Read the model definition and answer for the solid it produces. Units are mm, in the model's axes. A direction names the side the tool comes from. Coordinates: 2 decimals unless noted, no trailing zeros. Write each loop counter-clockwise with the first axis right and the second up, starting at its lowest first coordinate (ties: lowest second). Pieces come first, ordered by that corner, then holes.
(1) Given pin 1 (1.5 mm diameter, centred on y = 37, z = -7, fed in from -X); pin 2 (4.5 mm diameter, centred on y = 35.5, z = -2.5, fed in from +X); pin 3 (5 mm diameter, centred on y = 35, z = 0, fed in from +X) (3 decimals); pin 4 (1.5 mm diameter, centred on x = -35.5, y = 24.5, fed in from +Z), each flat-ended and moving along its own axis, determine where each tip first touches the part or whether it passes through.
(2) Which of the six approach directions +Z, -Z, +X, -X, +Y, -Y give full straight-line access (tool end or side, diameter ignored) to faces 1 (the flat face through (-17.091, 22.918, 29.392)), 2 (the flat face through (-11.7, 31.77, 26.73)), 3 (the flat face through (37, 25, 7.5)), 4 (the flat face through (-24.763, 24.86, -27.89)), 5 (the flat face through (29, 32, -3))?
(3) The mould has two halves that part along Z. Classify faces 6 (the flat face through (19.409, 25.887, 33.827)), 7 (the flat face through (-39, 26, 0)), 8 (the flat face through (-31.961, 7.605, 24.226)): +Z half, -Z half, draft (parallel to the pull), parting line (faces both ways), or undercut.
(4) Section A-A on z = 0 is taken. Write down the section's boundary in (x, y).
(5) Section B-B on y = 5 is taken. Write down the section's boundary in (x, z).
(6) Find the intervals of material crossed by probe 1 along Y at (x, z) = (31.5, 0); probe 2 along X at (y, z) = (32, 29.5); probe 3 along X at (y, z) = (38, 6.5), in increasing order.
(7) Section C-C on x = 0 is taken. Write down the section's boundary in (y, z).
from build123d import *

# Parameters (mm, degrees)
SKETCH1_R           = 45
BOSS_EXTRUDE1_DEPTH = 15
CUT_EXTRUDE1_DEPTH  = 66.383484153
CIRPATTERN1_COUNT   = 3
SKETCH4_R           = 4
BOSS_EXTRUDE2_DEPTH = 5
SKETCH6_R           = 7.5
SKETCH6_R_2         = 4
BOSS_EXTRUDE3_DEPTH = 10
CIRPATTERN2_COUNT   = 6


with BuildPart() as part:
    # Sketch1 → Boss-Extrude1 (new body)
    with BuildSketch(Plane(origin=(0, 0, 0), x_dir=(1, 0, 0), z_dir=(0, 1, 0))):
        with Locations(Location((0, 0, 0), (0, 0, 270))):
            Circle(SKETCH1_R)
    extrude(amount=BOSS_EXTRUDE1_DEPTH)

    # Sketch2 → Cut-Extrude1 (cut, through all)
    with BuildSketch(Plane(origin=(0, 15, 0), x_dir=(1, 0, 0), z_dir=(0, 1, 0))):
        with BuildLine():
            Line((-5, 35), (-5, 44.72135955))
            ThreePointArc((-5, 44.72135955), (0, 45), (5, 44.72135955))
            Line((5, 44.72135955), (5, 35))
            ThreePointArc((5, 35), (0, 30), (-5, 35))
        make_face()
    cut_extrude1 = extrude(amount=-CUT_EXTRUDE1_DEPTH, mode=Mode.SUBTRACT)

    # CirPattern1: Cut-Extrude1 ×3 about axis
    cirpattern1_axis = Axis((0, 0, 0), (0, 1, 0))
    for i in range(1, CIRPATTERN1_COUNT):
        add(cut_extrude1.rotate(cirpattern1_axis, i * 360 / CIRPATTERN1_COUNT), mode=Mode.SUBTRACT)

    # Sketch4 → Boss-Extrude2 (add)
    with BuildSketch(Plane(origin=(39, 0, 0), x_dir=(0, 0, -1), z_dir=(1, 0, 0))):
        with BuildLine():
            Line((-7.5, 35), (-7.5, 15))
            Line((-7.5, 15), (7.5, 15))
            Line((7.5, 15), (7.5, 35))
            ThreePointArc((7.5, 35), (0, 42.5), (-7.5, 35))
        make_face()
        with Locations((0, 35)):
            Circle(SKETCH4_R, mode=Mode.SUBTRACT)
    boss_extrude2 = extrude(amount=-BOSS_EXTRUDE2_DEPTH)

    # Sketch6 → Boss-Extrude3 (add)
    with BuildSketch(Plane(origin=(39, 0, 0), x_dir=(0, 0, -1), z_dir=(1, 0, 0))):
        with Locations((0, 35)):
            Circle(SKETCH6_R)
        with Locations((0, 35)):
            Circle(SKETCH6_R_2, mode=Mode.SUBTRACT)
    boss_extrude3 = extrude(amount=-BOSS_EXTRUDE3_DEPTH)

    # CirPattern2: Boss-Extrude2, Boss-Extrude3 ×6 about axis
    cirpattern2_axis = Axis((0, 0, 0), (0, 1, 0))
    add([boss_extrude2.rotate(cirpattern2_axis, i * 360 / CIRPATTERN2_COUNT) for i in range(1, CIRPATTERN2_COUNT)])
    add([boss_extrude3.rotate(cirpattern2_axis, i * 360 / CIRPATTERN2_COUNT) for i in range(1, CIRPATTERN2_COUNT)])


solid = part.part
Response:
1. pin 1: stops at x = -39
1. pin 2: stops at x = 39
1. pin 3: passes through
1. pin 4: stops at z = 7.5
2. face 1: none
2. face 2: +Y
2. face 3: +Z, +X, -X, +Y
2. face 4: -X, +Y
2. face 5: +Z, -Z, +Y
3. face 6: +Z half
3. face 7: draft
3. face 8: undercut
4. outline: (-45, 0) - (45, 0) - (45, 15) - (39, 15) - (39, 31) - (29, 31) - (29, 27.5) - (34, 27.5) - (34, 15) - (-34, 15) - (-34, 27.5) - (-29, 27.5) - (-29, 31) - (-39, 31) - (-39, 15) - (-45, 15) - close; (-39, 39) - (-29, 39) - (-29, 42.5) - (-39, 42.5) - close; (29, 39) - (39, 39) - (39, 42.5) - (29, 42.5) - close
5. outline: (-41.23, 18.03) arc R45 ccw to (-5, -44.72) - (-5, -35) arc R5 cw to (5, -35) - (5, -44.72) arc R45 ccw to (41.23, 18.03) - (32.81, 13.17) arc R5 cw to (27.81, 21.83) - (36.23, 26.69) arc R45 ccw to (-36.23, 26.69) - (-27.81, 21.83) arc R5 cw to (-32.81, 13.17) - close
6. probe 1: y = 0 to 15, 27.5 to 31, 39 to 42.5
6. probe 2: x = -25.69 to -20.09, -13.98 to -9.09, 9.09 to 13.98, 20.09 to 25.69
6. probe 3: x = -39 to -29, 29 to 39
7. outline: (0, -30) - (15, -30) - (15, 45) - (0, 45) - close
